Answer from the drawing. Dimensions are ordinates in mm from the lowest x, y and z of the part. A direction names the side the tool comes from. Coordinates: 2 decimals unless noted, no trailing zeros. Write each loop counter-clockwise with the first axis right and the second up, starting at its lowest first coordinate (ties: lowest second). Pieces come first, ordered by that corner, then holes.
(1) The part is cut by section A-A, the plane y = 9.5. Determine the outline of the cut face in (x, z), and give its area (3 significant figures).
(2) The part is cut by section B-B, the plane x = 6. Determine the outline of the cut face in (y, z).
(3) Given pin 1 (3.5 mm diameter, centred on y = 9.5, z = 6, fed in from -X); pin 2 (6 mm diameter, centred on x = 7, z = 6.5, fed in from -Y); pin 3 (2.5 mm diameter, centred on y = 8.5, z = 5.5, fed in from +X); pin 4 (2 mm diameter, centred on x = 9, y = 1.5, fed in from +Z), each flat-ended and moving along its own axis, determine where each tip first touches the part or whether it passes through.
(4) Which of the six approach directions +Z, -Z, +X, -X, +Y, -Y give full straight-line access (tool end or side, diameter ignored) to the marked faces 1, 2, 3 and 4?
(5) Straight lines are drawn through the part: line 1 along X through (y, z) = (9.7, 6); line 2 along Y through (x, z) = (11, 5). For each, find the intervals that lie inside material, in ascending order.
(6) The part is cut by section D-D, the plane y = 3.25. Determine the outline of the cut face in (x, z), and give its area (3 significant figures).
(7) Determine the mould class of the marked faces 5, 6 and 7 for opening direction X: pulls with the +X half, pulls with the -X half, needs draft (parallel to the pull), parting line crosses it, or undercut.
(8) The part is cut by section C-C, the plane z = 6. Determine the outline of the cut face in (x, y), and give its area (3 significant figures).
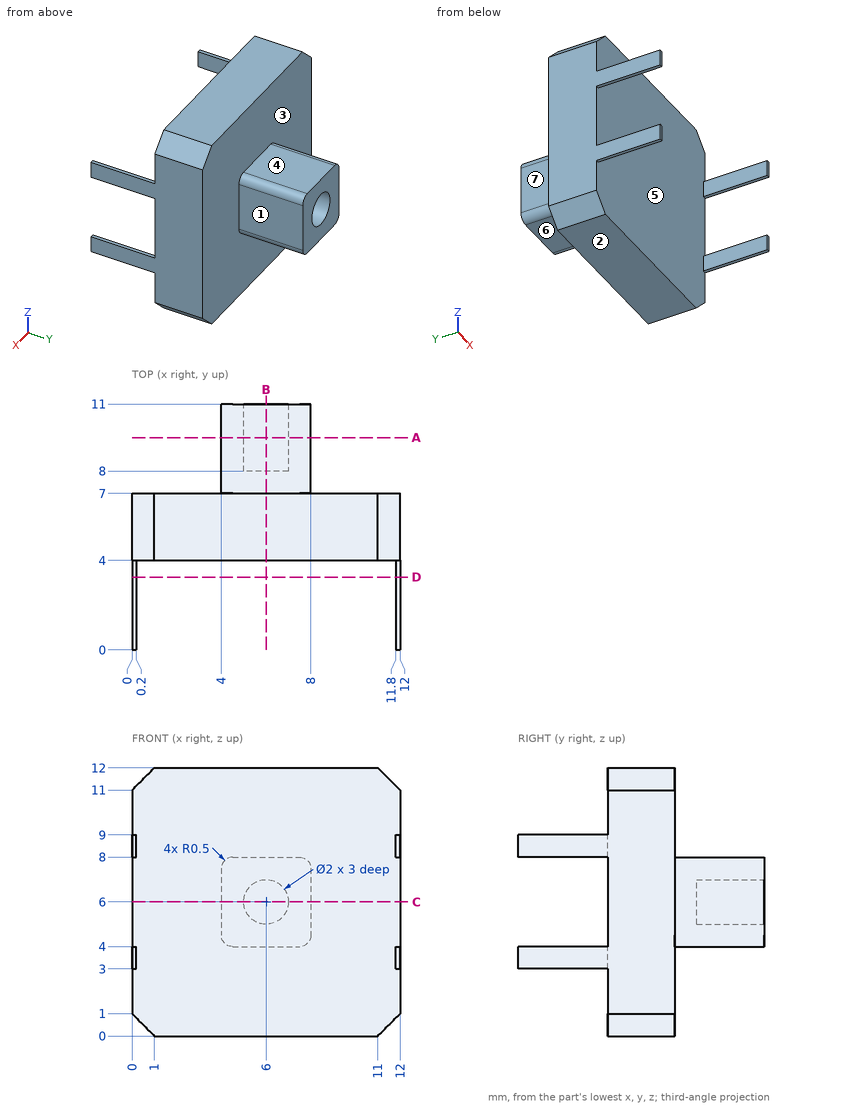
Computed:
1. outline: (4, 4.5) arc R0.5 ccw to (4.5, 4) - (7.5, 4) arc R0.5 ccw to (8, 4.5) - (8, 7.5) arc R0.5 ccw to (7.5, 8) - (4.5, 8) arc R0.5 ccw to (4, 7.5) - close; hole circle Ø2 at (6, 6)
1. area: 12.6 mm2
2. outline: (4, 0) - (7, 0) - (7, 4) - (11, 4) - (11, 5) - (8, 5) - (8, 7) - (11, 7) - (11, 8) - (7, 8) - (7, 12) - (4, 12) - close
3. pin 1: stops at x = 4
3. pin 2: stops at y = 4
3. pin 3: stops at x = 8
3. pin 4: passes through
4. face 1: +Z, -Z, +X, +Y
4. face 2: -Z, +X, -X, +Y, -Y
4. face 3: +Y
4. face 4: +Z, +X, -X, +Y
5. line 1: x = 4 to 5, 7 to 8
5. line 2: y = 4 to 7
6. outline: (0, 3) - (0.2, 3) - (0.2, 4) - (0, 4) - close; (0, 8) - (0.2, 8) - (0.2, 9) - (0, 9) - close; (11.8, 3) - (12, 3) - (12, 4) - (11.8, 4) - close; (11.8, 8) - (12, 8) - (12, 9) - (11.8, 9) - close
6. area: 0.800 mm2
7. face 5: undercut
7. face 6: needs draft
7. face 7: pulls with the -X half
8. outline: (0, 4) - (12, 4) - (12, 7) - (8, 7) - (8, 11) - (7, 11) - (7, 8) - (5, 8) - (5, 11) - (4, 11) - (4, 7) - (0, 7) - close
8. area: 46.0 mm2
